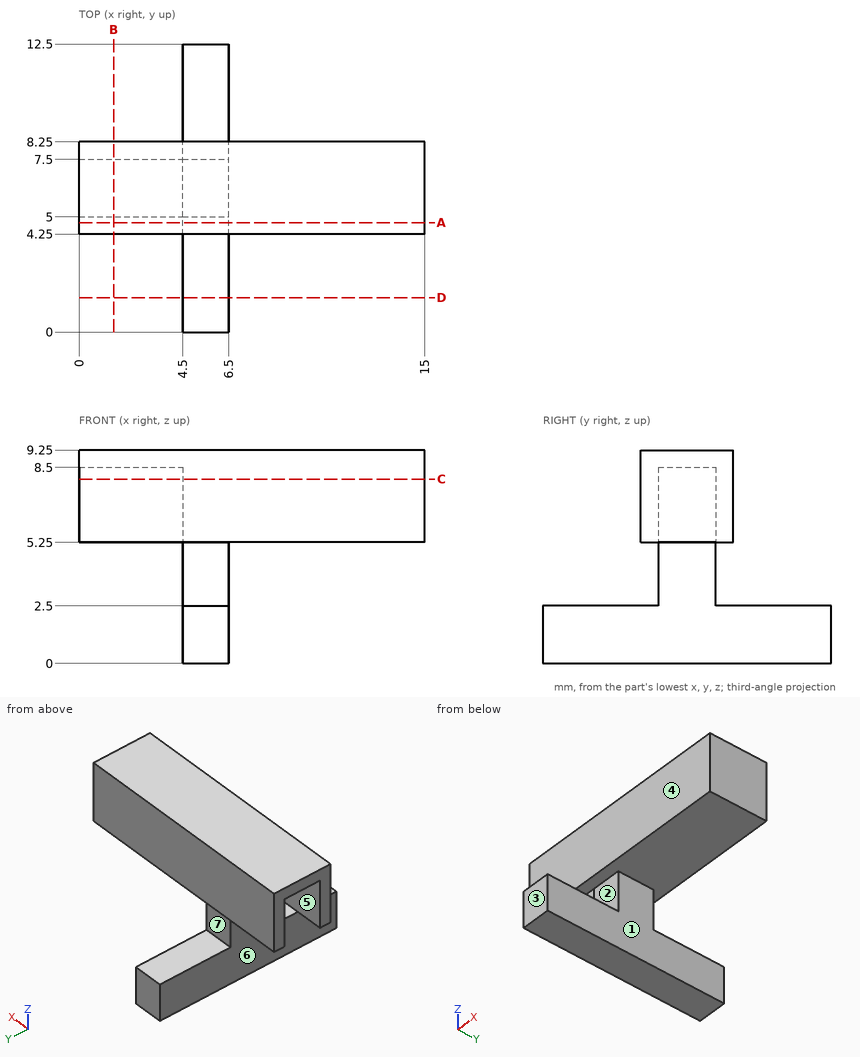
Check sheet for the drawn part. Datum: minimum x, y, z corner. Units: mm. A direction names the side the tool comes from. Round coordinates to 2 decimals unless told otherwise and drop trailing zeros. Order: outer loops, then holes, each group sorted by start corner. A loop starts at its lowest first (then second) coordinate and runs counter-clockwise, first axis right, second up.
1) Section check D-D (y = 1.5). Record the boundary of the cut face in (x, z).
2) Go/stop test with flat-tipped pins: pin 1 Ø1 at (x, z) = (5.5, 4) entering from +Y; pin 2 Ø1.2 at (x, z) = (5.5, 7) entering from +Y; pin 3 Ø1 at (x, z) = (2, 6) entering from -Y. Record where each tip stops, or that it passes through.
3) Section check A-A (y = 4.75). Record the boundary of the cut face in (x, z).
4) Tool access check on the marked faces 1, 2 and 3. Record the directions out of +Z, -Z, +X, -X, +Y, -Y that give a thin tool (end or side, any length) a straight path to the whole face; none if there is none.
5) Section check B-B (x = 1.5). Record the boundary of the cut face in (y, z).
6) Scan lines: line 1 (X direction, y = 10.5, z = 2); line 2 (Y direction, x = 11.75, z = 7.75); line 3 (Z direction, x = 14, y = 4.75). Record each from-to range of solid material in increasing order.
7) Mould release check, pull along Y, two halves, no side actions. Record for the marked faces 4, 5, 6 and 7: +Y half, -Y half, draft (parallel to the pull), parting line (faces both ways), or undercut.
8) Section check C-C (z = 8). Record the boundary of the cut face in (x, y).
Result:
1. outline: (4.5, 0) - (6.5, 0) - (6.5, 2.5) - (4.5, 2.5) - close
2. pin 1: stops at y = 7.5
2. pin 2: stops at y = 8.25
2. pin 3: stops at y = 4.25
3. outline: (0, 5.25) - (15, 5.25) - (15, 9.25) - (0, 9.25) - close; (4.5, 0) - (6.5, 0) - (6.5, 2.5) - (4.5, 2.5) - close
4. face 1: -Z, +X, +Y, -Y
4. face 2: +X, -X, -Y
4. face 3: +Z, -Z, +X, -X, -Y
5. outline: (4.25, 5.25) - (5, 5.25) - (5, 8.5) - (7.5, 8.5) - (7.5, 5.25) - (8.25, 5.25) - (8.25, 9.25) - (4.25, 9.25) - close
6. line 1: x = 4.5 to 6.5
6. line 2: y = 4.25 to 8.25
6. line 3: z = 5.25 to 9.25
7. face 4: -Y half
7. face 5: undercut
7. face 6: undercut
7. face 7: +Y half
8. outline: (0, 4.25) - (15, 4.25) - (15, 8.25) - (0, 8.25) - (0, 7.5) - (4.5, 7.5) - (4.5, 5) - (0, 5) - close
